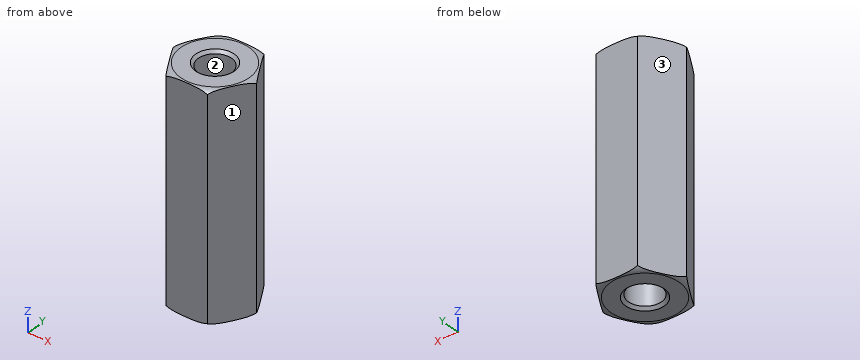
```python
from build123d import *

# Parameters (mm, degrees)
BOSS_EXTRUDE2_DEPTH     = 20
CUT_EXTRUDE5_DEPTH      = 21.606936666
CUT_EXTRUDE5_DEPTH_BACK = 21.606936666
SKETCH2_R               = 1.5
CHAMFER1_SIZE           = 0.25


with BuildPart() as part:
    # Sketch3 → Boss-Extrude2 (new body)
    with BuildSketch(Plane.XY):
        Polygon((3.75277675, 0), (1.876388375, 3.25), (-1.876388375, 3.25), (-3.75277675, 0), (-1.876388375, -3.25), (1.876388375, -3.25), align=None)
    extrude(amount=BOSS_EXTRUDE2_DEPTH)

    # Sketch5 → Cut-Revolve1 (revolve, cut)
    with BuildSketch(Plane(origin=(0, 0, 0), x_dir=(0, 0, -1), z_dir=(1, 0, 0))):
        with BuildLine():
            Line((-20, 0), (-20, 3.1))
            ThreePointArc((-20, 3.1), (-19.707106781, 3.807106781), (-19, 4.1))
            Line((-19, 4.1), (-1, 4.1))
            ThreePointArc((-1, 4.1), (-0.292893219, 3.807106781), (0, 3.1))
            Line((0, 3.1), (0, 1.684209227))
            Line((0, 1.684209227), (1.086869428, 1.684209227))
            Line((1.086869428, 1.684209227), (1.086869428, 4.997067517))
            Line((1.086869428, 4.997067517), (-20.5, 4.997067517))
            Line((-20.5, 4.997067517), (-20.5, 0))
            Line((-20.5, 0), (-20, 0))
        make_face()
    revolve(axis=Axis((0, 0, 20), (0, 0, 1)), mode=Mode.SUBTRACT)

    # Sketch2 → Cut-Extrude5 (cut, two sides: drawn at the far end of the back side and taken through both)
    with BuildSketch(Plane.XY.offset(-CUT_EXTRUDE5_DEPTH_BACK)):
        Circle(SKETCH2_R)
    extrude(amount=CUT_EXTRUDE5_DEPTH + CUT_EXTRUDE5_DEPTH_BACK, mode=Mode.SUBTRACT)

    # Chamfer1
    chamfer1_edges = [part.edges().sort_by_distance(p)[0] for p in [
        (-1.5, 0, 0),
        (-1.5, 0, 20),
    ]]
    chamfer(chamfer1_edges, length=CHAMFER1_SIZE)


solid = part.part
```
The listing builds one solid part. Answer for the finished solid, in the listing's coordinates (mm). Face numbers are marked on the shaded views. Give positions to 0.01 mm unless a question says otherwise; leave off trailing zeros. Order: outer loops, then holes, each group sorted by start corner. A loop starts at its lowest first (then second) coordinate and runs counter-clockwise, first axis right, second up. Notation, with made-up numbers: (13, -9.75) -> (66, -9.75) arc R26 cw to (66, 18.25) -> close; hole circle Ø1 at (53.5, -34). An arc over 180 degrees is marked (long way). Answer as a JSON object with one key per item and string values. Group by question number.
Item 1: Consider L1, parallel to Y at x = 0, z = 7.25; L2, parallel to X at y = -1.25, z = 4.5; L3, parallel to Y at x = -0.75, z = 18.5. Determine where each line is inside the solid, lowest interval first. Write a range as from..to.
Item 2: The part is cut by section A-A on x = 0. Write down the section's boundary in (y, z).
Item 3: The part is cut by section B-B on z = 16.5. Write down the section's boundary in (x, y), and give its area (3 significant figures).
Item 4: Determine the mould class of the marked faces 1, 2 and 3 for opening direction Y: pulls with the +Y half, pulls with the -Y half, needs draft (parallel to the pull), parting line crosses it, or undercut.
Item 5: A flat-ended cylindrical pin translates along its axis: pin 1 (3 mm diameter, centred on x = -0.5, y = -1, fed in from -Z). Find the tip coordinate at first contact, or state that the pin passes through.
Result set:
{
 "1": {"L1": "-3.25..-1.5, 1.5..3.25", "L2": "-3.03..-0.83, 0.83..3.03", "L3": "-3.25..-1.3, 1.3..3.25"},
 "2": {"outline": "(-3.25, 0.01) arc R1 ccw to (-3.1, 0) -> (-1.75, 0) -> (-1.5, 0.25) -> (-1.5, 19.75) -> (-1.75, 20) -> (-3.1, 20) arc R1 ccw to (-3.25, 19.99) -> close; (1.5, 0.25) -> (1.75, 0) -> (3.1, 0) arc R1 ccw to (3.25, 0.01) -> (3.25, 19.99) arc R1 ccw to (3.1, 20) -> (1.75, 20) -> (1.5, 19.75) -> close"},
 "3": {"outline": "(-3.75, 0) -> (-1.88, -3.25) -> (1.88, -3.25) -> (3.75, 0) -> (1.88, 3.25) -> (-1.88, 3.25) -> close; hole circle Ø3 at (0, 0)", "area": "29.5 mm²"},
 "4": {"face 1": "pulls with the -Y half", "face 2": "undercut", "face 3": "pulls with the +Y half"},
 "5": {"pin 1": "z = 0"}
}
